Geometry: final body of the model. Coordinates: model frame, mm. Give positions to 0.01 mm unless a question says otherwise; leave off trailing zeros. Write each loop counter-clockwise with the first axis right and the second up, starting at its lowest first coordinate (ties: lowest second). Pieces come first, ordered by that corner, then holes.
Autodesk Inventor part; units mm, degrees
ref_plane "YZ Plane" through (0, 0, 0) normal (1, 0, 0) x (0, 1, 0)
ref_plane "XZ Plane" through (0, 0, 0) normal (0, 1, 0) x (-1, 0, 0)
ref_plane "XY Plane" through (0, 0, 0) normal (0, 0, 1) x (1, 0, 0)
sketch "스케치1" plane through (0, 0, 0) normal (0, 0, 1) x (1, 0, 0)
  circle A0 centre (0, 0) radius 0.4
  circle A1 centre (0, 0) radius 0.5
  line L0 (0, 0.5) -> (7.6, 0.5)
  line L1 (7.6, 0.5) -> (7.6, -0.5)
  line L2 (7.6, -0.5) -> (0, -0.5)
  line L3 (0, -0.5) -> (0, 0.5)
  point P0 (0, -0.5)
  dimension "d1" = 1
  dimension "d0" = 0.8
  dimension "d2" = 1
  dimension "d7" = 7.6
extrude "돌출1" add sketch "스케치1" along normal mid plane 4 contours A0 L3 | L3 A0
extrude "돌출2" add sketch "스케치1" along normal mid plane 1.8 contours A0 L3 A1 | A0 L3 A1 | L0 L1 L2 A1
fillet "모깎기1" radius 0.1 2 edges at (7.6, 0.5, 0) (7.6, -0.5, 0)
properties part number "집게 고정"
Q1. Section C-C on z = -1.2. Output: boundary loops of the cut face in (x, y), plus the area to 3 significant figures.
Filled sheet:
outline: circle Ø0.8 at (0, 0)
area: 0.503 mm2
Q2. Ray query, line 1 along Z through (x, y) = (1.5, 0.2); line 2 along X through (y, z) = (0.3, -0.25); line 3 along X through (y, z) = (-0.2, -0.4). Return the intervals inside material, ascending.
Filled sheet:
line 1: z = -0.9 to 0.9
line 2: x = -0.4 to 7.6
line 3: x = -0.46 to 7.6
Q3. Section A-A on y = 0. Output: boundary loops of the cut face in (x, z), plus the area to 3 significant figures.
Filled sheet:
outline: (-0.5, -0.9) - (-0.4, -0.9) - (-0.4, -2) - (0.4, -2) - (0.4, -0.9) - (7.6, -0.9) - (7.6, 0.9) - (0.4, 0.9) - (0.4, 2) - (-0.4, 2) - (-0.4, 0.9) - (-0.5, 0.9) - close
area: 16.3 mm2
Q4. Section B-B on x = 1.25. Output: boundary loops of the cut face in (y, z).
Filled sheet:
outline: (-0.5, -0.9) - (0.5, -0.9) - (0.5, 0.9) - (-0.5, 0.9) - close
